The model under review builds one solid part; all positions refer to its coordinate system, in mm. Face numbers are marked on the shaded views. A direction names the side the tool comes from. Coordinates: 2 decimals unless noted, no trailing zeros. Loops run counter-clockwise (first coordinate to the right, second up) from the corner with the lowest first, then second, coordinate; pieces in that order, holes last. Notation, with made-up numbers: (-39.75, 31.5) -> (9.25, 31.5) arc R6 cw to (9.25, 35.5) -> close; hole circle Ø11 at (-29, 12). An arc over 180 degrees is marked (long way). One line per question, with ' | ' between items. Start each with the question number.
from build123d import *
from OCP.BRepFilletAPI import BRepFilletAPI_MakeChamfer

# Parameters (mm, degrees)
SKETCH4_W                = 12.46
SKETCH4_H                = 17.25
BOSS_EXTRUDE3_DEPTH      = 6
BOSS_EXTRUDE6_DEPTH      = 7.3
BOSS_EXTRUDE6_DEPTH_BACK = 17.25
SKETCH8_R                = 12.546781182
SKETCH8_R_2              = 11.15
BOSS_EXTRUDE4_DEPTH      = 17.25
SKETCH6_R                = 2
CUT_EXTRUDE1_DEPTH       = 5
CHAMFER1_SIZE            = 0.5
CHAMFER1_SIZE_2          = 0.866025404
SKETCH10_W               = 12.46
SKETCH10_H               = 23.7
CUT_EXTRUDE3_DEPTH       = 17.25
CUT_EXTRUDE4_REACH       = 83.955
SKETCH11_W               = 5
SKETCH11_H               = 3
BOSS_EXTRUDE7_START      = -7.3
BOSS_EXTRUDE7_DEPTH      = 7.3


with BuildPart() as part:
    # Sketch4 → Boss-Extrude3 (new body)
    with BuildSketch(Plane.XY):
        with Locations((0, 63.875025481)):
            Rectangle(SKETCH4_W, SKETCH4_H)
    extrude(amount=BOSS_EXTRUDE3_DEPTH)



with BuildPart() as body_2:
    # Sketch8 → Boss-Extrude6 (new, two sides: drawn at the far end of the back side and taken through both)
    with BuildSketch(Plane(origin=(0, 55.250025481, 0), x_dir=(-1, 0, 0), z_dir=(0, -1, 0)).offset(-BOSS_EXTRUDE6_DEPTH_BACK)):
        with Locations(Location((0, -23.55, 0), (0, 0, 90))):
            Circle(SKETCH8_R)
        with Locations(Location((0, -23.55, 0), (0, 0, 90))):
            Circle(SKETCH8_R_2, mode=Mode.SUBTRACT)
    extrude(amount=BOSS_EXTRUDE6_DEPTH + BOSS_EXTRUDE6_DEPTH_BACK)


with BuildPart() as part_1:
    add(part.part)

    add(body_2.part)  # Boss-Extrude4 merges body 2
    # Sketch5 → Boss-Extrude4 (add)
    with BuildSketch(Plane(origin=(0, 72.500025481, 0), x_dir=(1, 0, 0), z_dir=(0, 1, 0))):
        with BuildLine():
            Line((12.546781182, -23.55), (12.546781182, 0))
            Line((12.546781182, 0), (6.23, 0))
            Line((6.23, 0), (6.23, -29.7))
            Line((6.23, -29.7), (-6.23, -29.7))
            Line((-6.23, -29.7), (-6.23, 0))
            Line((-6.23, 0), (-12.546781182, 0))
            Line((-12.546781182, 0), (-12.546781182, -23.55))
            ThreePointArc((-12.546781182, -23.55), (0, -36.096781182), (12.546781182, -23.55))
        make_face()
    extrude(amount=-BOSS_EXTRUDE4_DEPTH)

    # Sketch6 → Cut-Extrude1 (cut)
    with BuildSketch(Plane(origin=(0, 72.500025481, 0), x_dir=(1, 0, 0), z_dir=(0, 1, 0))):
        with Locations(Location((0, -3.5, 0), (0, 0, 270))):
            Circle(SKETCH6_R)
        with Locations(Location((0, -32.2, 0), (0, 0, 270))):
            Circle(SKETCH6_R)
    extrude(amount=-CUT_EXTRUDE1_DEPTH, mode=Mode.SUBTRACT)

    # Chamfer1
    chamfer1_edges_1 = [part_1.edges().sort_by_distance(p)[0] for p in [
        (0, 72.500025481, 1.5),
    ]]
    chamfer1_side_1 = [part_1.faces().sort_by_distance(p)[0] for p in [
        (0, 72.500025481, 1.49),
    ]]
    chamfer1_edges_2 = [part_1.edges().sort_by_distance(p)[0] for p in [
        (0, 72.500025481, 30.2),
    ]]
    chamfer1_side_2 = [part_1.faces().sort_by_distance(p)[0] for p in [
        (0, 72.500025481, 30.19),
    ]]
    chamfer1 = BRepFilletAPI_MakeChamfer(part_1.part.solid().wrapped)
    for e in chamfer1_edges_1:
        chamfer1.Add(CHAMFER1_SIZE - 0.0001, CHAMFER1_SIZE_2 - 0.0001, e.wrapped, chamfer1_side_1[0].wrapped)
    for e in chamfer1_edges_2:
        chamfer1.Add(CHAMFER1_SIZE - 0.0001, CHAMFER1_SIZE_2 - 0.0001, e.wrapped, chamfer1_side_2[0].wrapped)
    add(Compound.cast(chamfer1.Shape()), mode=Mode.REPLACE)  # a hair under: the kernel refuses the full size

    # Sketch10 → Cut-Extrude3 (cut)
    with BuildSketch(Plane(origin=(0, 72.500025481, 0), x_dir=(1, 0, 0), z_dir=(0, 1, 0))):
        with Locations((0, -17.85)):
            Rectangle(SKETCH10_W, SKETCH10_H)
    extrude(amount=-CUT_EXTRUDE3_DEPTH, mode=Mode.SUBTRACT)

    # Sketch11 → Cut-Extrude4 (cut, up to next)
    with BuildSketch(Plane.XY.offset(36.096781182), mode=Mode.PRIVATE) as cut_extrude4_sk1:
        with Locations((0, 56.750025481)):
            Rectangle(SKETCH11_W, SKETCH11_H)
    cut_extrude4_tool1 = extrude(cut_extrude4_sk1.sketch, amount=-CUT_EXTRUDE4_REACH, mode=Mode.PRIVATE) & part_1.part
    add(cut_extrude4_tool1.solids().sort_by_distance((0, 56.750025, 36.096781))[0], mode=Mode.SUBTRACT)

    # Sketch13 → Boss-Extrude7 (add)
    with BuildSketch(Plane.XZ.offset(-47.950025481).offset(BOSS_EXTRUDE7_START)):
        with BuildLine():
            Line((-12.546781182, 23.55), (-12.546781182, 0))
            Line((-12.546781182, 0), (12.546781182, 0))
            Line((12.546781182, 0), (12.546781182, 23.55))
            ThreePointArc((12.546781182, 23.55), (0, 11.003218818), (-12.546781182, 23.55))
        make_face()
    extrude(amount=BOSS_EXTRUDE7_DEPTH)


solid = part_1.part
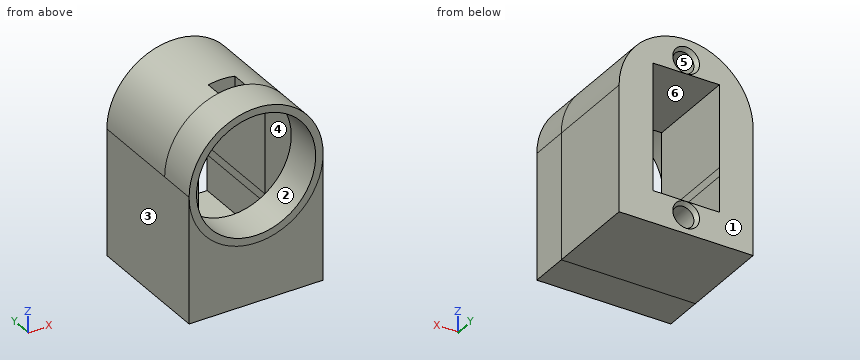
1) Wall thickness on L1, parallel to X at y = 58.5, z = 15; L2, parallel to Z at x = -2.5, y = 61.25; L3, parallel to X at y = 69.25, z = 3.5: over which ranges is each line inside the solid? List them lowest first.
2) Consider section B-B, the plane y = 67. Write out the cut boundary in (x, z), plus the area to 3 significant figures.
3) Consider section D-D, the plane z = 3.5. Write out the cut boundary in (x, y), plus the area to 3 significant figures.
4) Consider section C-C, the plane x = 3.5. Write out the cut boundary in (y, z).
5) Mouldability with a two-part tool opening along X and no side actions: class the marked faces 1, 2 and 3 as +X half, -X half, draft (parallel to the pull), parting line (faces both ways), or undercut.
6) Insertion check: pin 1 Ø1 at (x, y) = (9.5, 51) entering from +Z; pin 2 Ø5.5 at (x, z) = (-0.5, 31.5) entering from -Y; pin 3 Ø4 at (x, z) = (-3.5, 21) entering from -Y; pin 4 Ø1.2 at (x, z) = (0, 3.5) entering from +Y. Each pin has a flat end and moves straight along its axis. Give the tip position at first contact, or say it passes through.
7) Machinability: for the marked faces 4, 5 and 6, which of the approach directions +Z, -Z, +X, -X, +Y, -Y give a long, thin tool a straight path to every point of the face, cutting with its end or side? Answer none if there is none.
8) Consider section A-A, the plane x = 0. Give the number of separate pieces and of enclosed holes in the cut face, plus the area to 3 significant figures.
Filled sheet:
1) L1: -12.55 to -6.23, 6.23 to 12.55 | L2: 0 to 6, 29.7 to 35.85 | L3: -12.55 to -2, 2 to 12.55
2) outline: (-12.55, 0) -> (12.55, 0) -> (12.55, 23.55) arc R12.55 ccw to (-12.55, 23.55) -> close; hole (-6.23, 6) -> (6.23, 6) -> (6.23, 29.7) -> (-6.23, 29.7) -> close | area: 543 mm^2
3) outline: (-12.55, 47.95) -> (12.55, 47.95) -> (12.55, 72.5) -> (2.5, 72.5) -> (2, 71.63) -> (2, 67.5) -> (-2, 67.5) -> (-2, 71.63) -> (-2.5, 72.5) -> (-12.55, 72.5) -> close | area: 596 mm^2
4) outline: (47.95, 0) -> (72.5, 0) -> (72.5, 6) -> (55.25, 6) -> (55.25, 12.96) -> (47.95, 12.96) -> close; (47.95, 34.14) -> (55.25, 34.14) -> (55.25, 29.7) -> (72.5, 29.7) -> (72.5, 35.6) -> (47.95, 35.6) -> close
5) face 1: draft | face 2: undercut | face 3: -X half
6) pin 1: z = 32.29 | pin 2: y = 55.25 | pin 3: through | pin 4: y = 67.5
7) face 4: -Y | face 5: +Y | face 6: +Y, -Y
8) separate pieces: 3 | enclosed holes: 0 | area: 255 mm^2
